```python
from build123d import *

# Parameters (mm, degrees)
EXTRUSION1_DEPTH = 294.5
ESQUISSE2_R      = 1.5
EXTRUSION2_DEPTH = 300
ESQUISSE3_R      = 1.5
ESQUISSE3_R_2    = 2
EXTRUSION3_DEPTH = 300
ESQUISSE4_W      = 1.5
ESQUISSE4_H      = 20
EXTRUSION4_DEPTH = 5
ESQUISSE5_R      = 1.5
EXTRUSION5_DEPTH = 5


with BuildPart() as part:
    # Esquisse1 → Extrusion1 (new body)
    with BuildSketch(Plane.XY):
        Polygon((-17.43168638, 4.773368421), (-17.43168638, -15.226631579), (2.56831362, -15.226631579), (2.56831362, -13.726631579), (-15.93168638, -13.726631579), (-15.93168638, 4.773368421), align=None)
    extrude(amount=EXTRUSION1_DEPTH)

    # Esquisse2 → Extrusion2 (cut)
    with BuildSketch(Plane(origin=(0, -13.726631579, 0), x_dir=(-1, 0, 0), z_dir=(0, 1, 0))):
        with Locations((7.43168638, 8.5)):
            Circle(ESQUISSE2_R)
    extrude(amount=-EXTRUSION2_DEPTH, mode=Mode.SUBTRACT)

    # Esquisse3 → Extrusion3 (cut)
    with BuildSketch(Plane(origin=(-15.93168638, 0, 0), x_dir=(0, 0, -1), z_dir=(1, 0, 0))):
        with Locations((-8.5, -5.226631579)):
            Circle(ESQUISSE3_R)
        with Locations((-35, -7.726631579)):
            Circle(ESQUISSE3_R_2)
        with Locations((-46, -7.726631579)):
            Circle(ESQUISSE3_R_2)
        with Locations((-290, -7.726631579)):
            Circle(ESQUISSE3_R_2)
        with Locations((-279, -7.726631579)):
            Circle(ESQUISSE3_R_2)
        with Locations((-235, -5.226631579)):
            Circle(ESQUISSE3_R)
        with Locations((-90, -5.226631579)):
            Circle(ESQUISSE3_R)
    extrude(amount=-EXTRUSION3_DEPTH, mode=Mode.SUBTRACT)

    # Esquisse4 → Extrusion4 (add)
    with BuildSketch(Plane.XY.offset(294.5)):
        with Locations((-16.68168638, -5.226631579)):
            Rectangle(ESQUISSE4_W, ESQUISSE4_H)
    extrude(amount=EXTRUSION4_DEPTH)

    # Esquisse5 → Extrusion5 (cut)
    with BuildSketch(Plane.XZ.offset(15.226631579)):
        with Locations(Location((-9.93168638, 287, 0), (0, 0, 270))):
            Circle(ESQUISSE5_R)
    extrude(amount=-EXTRUSION5_DEPTH, mode=Mode.SUBTRACT)


solid = part.part
```
CAD build for the part. Positions are in the model's coordinates, mm. A direction names the side the tool comes from. Give positions to 0.01 mm unless a question says otherwise; leave off trailing zeros. Write each loop counter-clockwise with the first axis right and the second up, starting at its lowest first coordinate (ties: lowest second). Pieces come first, ordered by that corner, then holes. Notation, with made-up numbers: M 23,46.25 L 49,46.25 A15 ccw 49,64.25 Z; hole C 41.25,40.5 d3. An arc over 180 degrees is marked long. Return JSON: item names as keys, results as strings. Group by question number.
(1) Band-saw the part on B-B (y = -0.5). Give the cut face in (x, z).
(2) Flat gauge pins, fed straight in: pin 1 Ø5 at (x, z) = (-9.93, 287) entering from -Y; pin 2 Ø5 at (y, z) = (-7.73, 35) entering from +X; pin 3 Ø1.5 at (x, z) = (-9.5, 90.5) entering from +Y; pin 4 Ø2.5 at (y, z) = (-5.23, 90) entering from +X. Where does each tip first touch, or does it go through?
(3) 3-axis set-ups, long thin cutter, end or side, ignore diameter. For faces 1 (the face through (-7, -13.727, 145)), 2 (the face through (-17.432, -5, 148)): which of +Z, -Z, +X, -X, +Y, -Y reach the whole face in a straight line?
(4) Band-saw the part on A-A (z = 248.5). Give the cut face in (x, y), and give its area (4 significant figures).
(5) Drill centre lines: L1, parallel to Y at x = -17.1, z = 8.5; L2, parallel to X at y = -14.3, z = 287; L3, parallel to Y at x = -16.4, z = 46. Where is each one in solid material? Low to high. Write a range as [from, to].
Entries:
{
 "1": {"outline": "M -17.43,0 L -15.93,0 L -15.93,299.5 L -17.43,299.5 Z"},
 "2": {"pin 1": "stops at y = -15.23", "pin 2": "stops at x = -15.93", "pin 3": "stops at y = -13.73", "pin 4": "passes through"},
 "3": {"face 1": "+Z, -Z, +X, +Y", "face 2": "+Z, -Z, -X, +Y, -Y"},
 "4": {"outline": "M -17.43,-15.23 L 2.57,-15.23 L 2.57,-13.73 L -15.93,-13.73 L -15.93,4.77 L -17.43,4.77 Z", "area": "57.75 mm^2"},
 "5": {"L1": "y = [-15.23, -6.73], [-3.73, 4.77]", "L2": "x = [-17.43, -11.43], [-8.43, 2.57]", "L3": "y = [-15.23, -9.73], [-5.73, 4.77]"}
}
